Autodesk Inventor part; units mm, degrees
ref_plane "YZ Plane" through (0, 0, 0) normal (1, 0, 0) x (0, 1, 0)
ref_plane "XZ Plane" through (0, 0, 0) normal (0, 1, 0) x (-1, 0, 0)
ref_plane "XY Plane" through (0, 0, 0) normal (0, 0, 1) x (1, 0, 0)
sketch "Sketch1" plane through (0, 0, 0) normal (0, 0, 1) x (1, 0, 0)
  line L0 (0, 0) -> (0.8, 0)
  line L1 (0.8, 0) -> (0.8, 2.625)
  line L2 (0.8, 2.625) -> (0, 2.625)
  line L3 (0, 2.625) -> (0, 0)
  line L4 (0.8, 0) -> (1.6, 0)
  line L5 (1.6, 0) -> (1.6, 3.625)
  line L6 (1.6, 3.625) -> (0.8, 3.625)
  line L7 (0.8, 3.625) -> (0.8, 0)
  line L8 (1.6, 0) -> (2.85, 0)
  line L9 (2.85, 0) -> (2.85, 4.2)
  line L10 (2.85, 4.2) -> (1.6, 4.2)
  line L11 (1.6, 4.2) -> (1.6, 0)
  line L12 (2.85, 0) -> (6.1, 0)
  line L13 (6.1, 0) -> (6.1, 3.35)
  line L14 (6.1, 3.35) -> (2.85, 3.35)
  line L15 (2.85, 3.35) -> (2.85, 0)
  dimension "d0" = 5.25
  dimension "d1" = 7.25
  dimension "d2" = 8.4
  dimension "d3" = 6.7
  dimension "d4" = 0.8
  dimension "d7" = 1.6
  dimension "d8" = 2.85
  dimension "d9" = 6.1
revolve "Revolution1" add sketch "Sketch1" angle 360 about axis through (0, 0, 0) along (1, 0, 0)
hole "Hole1" at (0, 0, 0) direction (1, 0, 0) diameter 3.6 end through all
properties part number "308-14" material "Polypropylene"
For this review, take the finished solid that the model builds, in its own axes (mm). A direction names the side the tool comes from. Round coordinates to 2 decimals unless told otherwise and drop trailing zeros. Write each loop counter-clockwise with the first axis right and the second up, starting at its lowest first coordinate (ties: lowest second). Pieces come first, ordered by that corner, then holes. Notation, with made-up numbers: (-30.5, 77) - (25.5, 77) arc R35 cw to (25.5, 112) - close; hole circle Ø5 at (12.25, 49). An arc over 180 degrees is marked (long way). Answer as CSV lines item,"result". Start each with the question number.
(1) Add section C-C, the plane x = 1.75. State the section outline as (y, z) points.
(2) Machinability: for faces 1 (the cylindrical face through (0.4, 2.5, -0.8)), 2 (the cylindrical face through (4.452, -3.347, -0.147)), 3 (the flat face through (6.1, 1.4, -1.4)), which of the approach directions +Z, -Z, +X, -X, +Y, -Y give a long, thin tool a straight path to every point of the face, cutting with its end or side? Answer none if there is none.
(3) Mouldability with a two-part tool opening along Y and no side actions: class faces 4 (the flat face through (2.85, -3, -2)), 5 (the cylindrical face through (2.216, 4.006, -1.262)), 6 (the cylindrical face through (3.093, -0.541, 1.717)) as +Y half, -Y half, draft (parallel to the pull), parting line (faces both ways), or undercut.
(4) For line 1 (Z direction, x = 5.5, y = 0); line 2 (Z direction, x = 1.5, y = 0) (3 decimals); line 3 (X direction, y = -2.25, z = 2), list the stretches that pass through material, from the lowest coordinate up.
(5) Add section A-A, the plane y = 0. State the section outline as (x, z) points (3 decimals).
(6) For pin 1 (3 mm diameter, centred on x = 5, y = 1.5, fed in from -Z); pin 2 (2 mm diameter, centred on x = 3, y = 2, fed in from -Z); pin 3 (2 mm diameter, centred on x = 4, y = -1, fed in from +Z); pin 4 (2 mm diameter, centred on y = 0, z = 0, fed in from -X), all flat-tipped, find the tip position at first contact; note any pin that passes through.
(7) Add section D-D, the plane y = -2.75. State the section outline as (x, z) points, plus the area to 3 significant figures.
From the geometry:
1,outline,"circle Ø8.4 at (0, 0); hole circle Ø3.6 at (0, 0)"
2,face 1,"-X"
2,face 2,"+X"
2,face 3,"+Z, -Z, +X, +Y, -Y"
3,face 4,"draft"
3,face 5,"parting line"
3,face 6,"undercut"
4,line 1,"z = -3.35 to -1.8, 1.8 to 3.35"
4,line 2,"z = -3.625 to -1.8, 1.8 to 3.625"
4,line 3,"x = 0.8 to 6.1"
5,outline,"(0, -2.625) - (0.8, -2.625) - (0.8, -3.625) - (1.6, -3.625) - (1.6, -4.2) - (2.85, -4.2) - (2.85, -3.35) - (6.1, -3.35) - (6.1, -1.8) - (0, -1.8) - close; (0, 1.8) - (6.1, 1.8) - (6.1, 3.35) - (2.85, 3.35) - (2.85, 4.2) - (1.6, 4.2) - (1.6, 3.625) - (0.8, 3.625) - (0.8, 2.625) - (0, 2.625) - close"
6,pin 1,"stops at z = -3.35"
6,pin 2,"stops at z = -4.08"
6,pin 3,"stops at z = 3.35"
6,pin 4,"passes through"
7,outline,"(0.8, -2.36) - (1.6, -2.36) - (1.6, -3.17) - (2.85, -3.17) - (2.85, -1.91) - (6.1, -1.91) - (6.1, 1.91) - (2.85, 1.91) - (2.85, 3.17) - (1.6, 3.17) - (1.6, 2.36) - (0.8, 2.36) - close"
7,area,"24.2 mm²"
